from build123d import *

# Parameters (mm, degrees)
SKIZZE1_W                       = 20
SKIZZE1_H                       = 20
AUFSATZ_LINEAR_AUSTRAGEN1_DEPTH = 300
SKIZZE2_R                       = 3
SCHNITT_LINEAR_AUSTRAGEN1_DEPTH = 301.83217913


with BuildPart() as part:
    # Skizze1 → Aufsatz-Linear austragen1 (new body)
    with BuildSketch(Plane(origin=(0, 0, 0), x_dir=(0, 0, -1), z_dir=(1, 0, 0))):
        Rectangle(SKIZZE1_W, SKIZZE1_H)
    extrude(amount=AUFSATZ_LINEAR_AUSTRAGEN1_DEPTH)

    # Skizze2 → Schnitt-Linear austragen1 (cut, through all)
    with BuildSketch(Plane(origin=(0, 10, 0), x_dir=(1, 0, 0), z_dir=(0, 1, 0))):
        with Locations(Location((10, 0, 0), (0, 0, 270))):
            Circle(SKIZZE2_R)
        with Locations(Location((114, 0, 0), (0, 0, 270))):
            Circle(SKIZZE2_R)
        with Locations(Location((202, 0, 0), (0, 0, 270))):
            Circle(SKIZZE2_R)
    extrude(amount=-SCHNITT_LINEAR_AUSTRAGEN1_DEPTH, mode=Mode.SUBTRACT)


solid = part.part
Could you check a few things on this model? Use its own coordinates, in mm. Round coordinates to 2 decimals unless told otherwise and drop trailing zeros. Order: outer loops, then holes, each group sorted by start corner. A loop starts at its lowest first (then second) coordinate and runs counter-clockwise, first axis right, second up. Notation, with made-up numbers: M 13,51 L 46,51 A25 cw 46,79 Z; hole C 30.25,68.5 d1. An arc over 180 degrees is marked long. One line per item, written item: value.
(1) If we mould it in two halves opening along X, with no side actions, what happens to faces 1 (the flat face through (0, 0, 0)), 2 (the cylindrical face through (117, 0, 0)), 3 (the cylindrical face through (10.9, 0.14, 2.86)), 4 (the flat face through (148, 10, 0))? For each: released by +X, released by -X, zero draft, split by the parting line, or undercut.
Ans:
face 1: released by -X
face 2: undercut
face 3: undercut
face 4: zero draft
(2) I'm going to push a flat-ended pin straight in: P1, Ø3.5, axis at x = 114, z = 0, coming from the +Y side. Where does the tip first touch, or does it pass through?
Ans:
P1: passes through
(3) Imagine slicing it at A-A (z = 0). Write out the boundary of the cut face in (x, y).
Ans:
outline: M 0,-10 L 7,-10 L 7,10 L 0,10 Z; M 13,-10 L 111,-10 L 111,10 L 13,10 Z; M 117,-10 L 199,-10 L 199,10 L 117,10 Z; M 205,-10 L 300,-10 L 300,10 L 205,10 Z
(4) Imagine slicing it at B-B (x = 114). Write out the boundary of the cut face in (y, z), and give its area (3 significant figures).
Ans:
outline: M -10,-10 L 10,-10 L 10,-3 L -10,-3 Z; M -10,3 L 10,3 L 10,10 L -10,10 Z
area: 280 mm^2
(5) I need wall thicknesses on line 1 along X through (y, z) = (1.75, 0); line 2 along Z through (x, y) = (202, 2); line 3 along X through (y, z) = (-4.5, 1). Which ranges of each line are inside material? Lowest first, please. Write a range as from..to.
Ans:
line 1: x = 0..7, 13..111, 117..199, 205..300
line 2: z = -10..-3, 3..10
line 3: x = 0..7.17, 12.83..111.17, 116.83..199.17, 204.83..300
